Verification items for the finished model (mm, model axes). Face numbers are marked on the shaded views. Give positions to 0.01 mm unless a question says otherwise; leave off trailing zeros. Write each loop counter-clockwise with the first axis right and the second up, starting at its lowest first coordinate (ties: lowest second). Pieces come first, ordered by that corner, then holes. Notation, with made-up numbers: (29.5, 36) -> (57.5, 36) arc R27 cw to (57.5, 59) -> close; hole circle Ø11 at (-0.5, 75.25). An arc over 180 degrees is marked (long way). Answer as CSV lines item,"result". Start each with the question number.
1) Sectioned sample at A-A on x = 0. Record the cut outline in (y, z), and give its area (3 significant figures).
2) Sectioned sample at B-B on z = 0. Record the cut outline in (x, y).
3) Sectioned sample at C-C on y = 1.25. Record the cut outline in (x, z).
4) Gauge pin test, flat ends, axial feed: pin 1 Ø6 at (y, z) = (-4.5, 3.5) entering from +X; pin 2 Ø12 at (x, z) = (-8.5, 6) entering from +Y; pin 3 Ø2 at (y, z) = (6.5, -2) entering from +X; pin 4 Ø6 at (x, z) = (8, 2) entering from -Y. Record the tip position at first contact, or that the pin passes through.
5) Sectioned sample at D-D on x = -5.5. Record the cut outline in (y, z), and give its area (3 significant figures).
6) Mould release check, pull along Z, two halves, no side actions. Record for the marked faces 1 and 2: released by +Z, released by -Z, zero draft, split by the parting line, or undercut.
7) Material ranges on L1, parallel to Z at x = 0, y = -0.75; L2, parallel to Z at x = 0, y = -3.5; L3, parallel to X at y = 2, z = 0, recorded low to high.
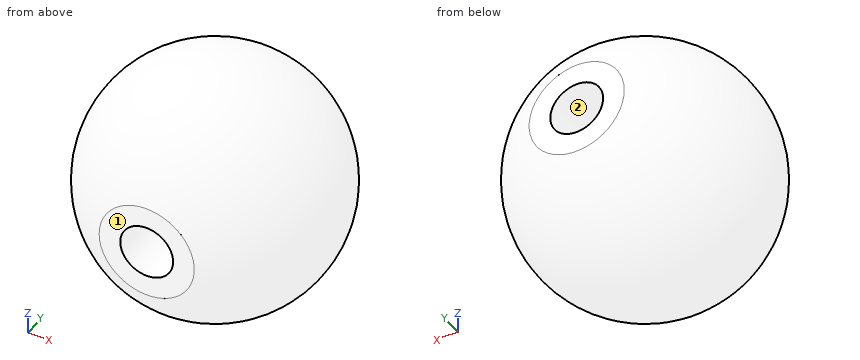
```python
from build123d import *

# Parameters (mm, degrees)
SKETCH2_R               = 2.5
CUT_EXTRUDE1_DEPTH      = 12.105084746
CUT_EXTRUDE1_DEPTH_BACK = 13.294915254
CUT_EXTRUDE2_DEPTH      = 12.7
CUT_EXTRUDE2_DEPTH_BACK = 12.7


with BuildPart() as part:
    # Sketch1 → Revolve1 (revolve)
    with BuildSketch(Plane.XY):
        with BuildLine():
            Line((0, 11.105084746), (0, -12.294915254))
            ThreePointArc((0, -12.294915254), (-11.7, -0.594915254), (0, 11.105084746))
        make_face()
    revolve(axis=Axis((0, 11.105084746, 0), (0, -1, 0)))

    # Sketch2 → Cut-Extrude1 (cut, two sides)
    with BuildSketch(Plane(origin=(0, 0, 0), x_dir=(1, 0, 0), z_dir=(0, 1, 0))) as cut_extrude1_sk:
        Circle(SKETCH2_R)
    extrude(amount=CUT_EXTRUDE1_DEPTH, mode=Mode.SUBTRACT)
    extrude(cut_extrude1_sk.sketch, amount=-CUT_EXTRUDE1_DEPTH_BACK, mode=Mode.SUBTRACT)

    # Sketch6 → Cut-Extrude2 (cut, two sides)
    with BuildSketch(Plane.XY) as cut_extrude2_sk:
        Polygon((0, 12.205084746), (-13.76858677, 12.205084746), (-13.76858677, 10.205084746), (12.631256699, 10.205084746), (12.631256699, 12.205084746), align=None)
        Polygon((0, -13.394915254), (12.631256699, -13.394915254), (12.631256699, -11.394915254), (-13.76858677, -11.394915254), (-13.76858677, -13.394915254), align=None)
    extrude(amount=CUT_EXTRUDE2_DEPTH, mode=Mode.SUBTRACT)
    extrude(cut_extrude2_sk.sketch, amount=-CUT_EXTRUDE2_DEPTH_BACK, mode=Mode.SUBTRACT)


solid = part.part
```
Ans:
1,outline,"(-11.39, -4.5) arc R11.7 ccw to (10.21, -4.5) -> (10.21, -2.5) -> (-11.39, -2.5) -> close; (-11.39, 2.5) -> (10.21, 2.5) -> (10.21, 4.5) arc R11.7 ccw to (-11.39, 4.5) -> close"
1,area,"311 mm²"
2,outline,"(-4.5, -11.39) -> (-2.5, -11.39) -> (-2.5, 10.21) -> (-4.5, 10.21) arc R11.7 ccw to start; (2.5, -11.39) -> (4.5, -11.39) arc R11.7 ccw to (4.5, 10.21) -> (2.5, 10.21) -> close"
3,outline,"circle Ø23.11 at (0, 0); hole circle Ø5 at (0, 0)"
4,pin 1,"stops at x = 11.48"
4,pin 2,"stops at y = 10.21"
4,pin 3,"stops at x = 9.81"
4,pin 4,"stops at y = -11.05"
5,outline,"circle Ø20.65 at (-0.59, 0)"
5,area,"335 mm²"
6,face 1,"zero draft"
6,face 2,"undercut"
7,L1,"z = -11.7 to -2.5, 2.5 to 11.7"
7,L2,"z = -11.33 to -2.5, 2.5 to 11.33"
7,L3,"x = -11.41 to -2.5, 2.5 to 11.41"
